Read the model definition and answer for the solid it produces. Units are mm, in the model's axes. A direction names the side the tool comes from. Round coordinates to 2 decimals unless told otherwise and drop trailing zeros. Order: outer loops, then holes, each group sorted by start corner. A loop starts at its lowest first (then second) coordinate and runs counter-clockwise, first axis right, second up. Notation, with made-up numbers: (-5.75, 13.25) - (29.25, 13.25) arc R26 ccw to (29.25, 35.25) - close; hole circle Ø10 at (17, 79). An arc over 180 degrees is marked (long way). Answer as a JSON object with one key per item and string values. Group by question number.
Q1. A cutting plane is placed at A-A on x = 0. Determine the outline of the cut face in (y, z), and give its area (3 significant figures).
Q2. A cutting plane is placed at D-D on x = 42. Determine the outline of the cut face in (y, z), and give its area (3 significant figures).
Q3. Consider line 1 (X direction, y = 280, z = -377.5); line 2 (Z direction, x = -130, y = 5.25); line 3 (Y direction, x = 130, z = -382). Determine where each line is inside the solid, lowest interval first.
Q4. A cutting plane is placed at B-B on x = -130. Count the separate pieces of the cut face and the enclosed holes in it, and give its area (3 significant figures).
Q5. Given pin 1 Ø18 at (x, y) = (-116.5, 283.5) entering from -Z; pin 2 Ø24 at (x, y) = (-130, 540) entering from -Z; pin 3 Ø1.5 at (y, z) = (152, -41) entering from -X; pin 4 Ø8 at (x, z) = (-28.5, -324) entering from +Y, each flat-ended and moving along its own axis, determine where each tip first touches the part or whether it passes through.
Q6. The mould has two halves that part along Z. Classify faces 1 (the flat face through (3, 0, 3)), 2 (the flat face through (-3, 25, -180)), 3 (the flat face through (-116, 10, 124)): pulls with the +Z half, pulls with the -Z half, needs draft (parallel to the pull), parting line crosses it, or undercut.
Q7. A tool of negligible diameter and unlimited length cuts with its end or side. For faces 4 (the flat face through (3, 230, -385)), 5 (the cylindrical face through (-136.503, 4.93, -159.287)), 6 (the cylindrical face through (100.03, 278.68, -405.07)), from which of +Z, -Z, +X, -X, +Y, -Y can it reach the whole face along a straight path? Write none if from no direction.
Solid Edge part; units mm, degrees
sketch "Sketch1" plane through (0, 0, 0) normal (1, 0, 0) x (0, 1, 0)
  line L0 (410, -260) -> (410, -410)
  line L1 (0, 0) -> (150, 0)
  arc A0 (150, 0) -> (410, -260) centre (150, -260) cw
sketch "Sketch2" plane through (0, 0, 0) normal (0, -1, 0) x (1, 0, 0)
  circle A0 centre (0, 0) radius 145
sweep "SweptProtrusion_1" add profiles "Sketch2" path "Sketch1"
sketch "Sketch3" plane through (0, 0, 0) normal (1, 0, 0) x (0, 1, 0)
  line L0 (410, -260) -> (410, -410)
  line L1 (0, 0) -> (150, 0)
  arc A0 (150, 0) -> (410, -260) centre (150, -260) cw
sketch "Sketch4" plane through (0, 0, 0) normal (0, -1, 0) x (1, 0, 0)
  circle A0 centre (0, 0) radius 130
sweep "SweptCutout_1" cut profiles "Sketch4" path "Sketch3"
sketch "Sketch5" plane through (0, 0, 0) normal (0, -1, 0) x (1, 0, 0)
  line L0 (180, 180) -> (-180, 180)
  line L1 (-180, 180) -> (-180, -180)
  line L2 (-180, -180) -> (180, -180)
  line L3 (180, -180) -> (180, 180)
  circle A0 centre (0, 0) radius 130
extrude "ExtrudedProtrusion_2" add sketch "Sketch5" against normal blind 50
sketch "Sketch6" plane through (0, 0, 0) normal (0, -1, 0) x (1, 0, 0)
  circle A0 centre (130, 130) radius 30
  circle A1 centre (-130, 130) radius 30
  circle A2 centre (-130, -130) radius 30
  circle A3 centre (130, -130) radius 30
extrude "ExtrudedCutout_1" cut sketch "Sketch6" against normal blind 10
sketch "Sketch7" plane through (0, 0, 0) normal (0, -1, 0) x (1, 0, 0)
  circle A0 centre (130, 130) radius 15
  circle A1 centre (-130, 130) radius 15
  circle A2 centre (-130, -130) radius 15
  circle A3 centre (130, -130) radius 15
extrude "ExtrudedCutout_2" cut sketch "Sketch7" against normal blind 50
mirror "Mirror1" about plane through (0, 333.8478, -76.1522) normal (0, -0.7071068, 0.7071068) of "ExtrudedProtrusion_2", "ExtrudedCutout_1", "ExtrudedCutout_2", "SweptProtrusion_1"
Result set:
{
 "1": {"outline": "(0, -180) - (50, -180) - (50, -145) - (150, -145) arc R115 cw to (265, -260) - (265, -360) - (230, -360) - (230, -410) - (590, -410) - (590, -360) - (555, -360) - (555, -260) arc R405 ccw to (150, 145) - (50, 145) - (50, 180) - (0, 180) - close", "area": "212,000 mm²"},
 "2": {"outline": "(0, -180) - (50, -180) - (50, -138.78) - (150, -138.78) arc R121.22 cw to (271.22, -260) - (271.22, -360) - (230, -360) - (230, -410) - (590, -410) - (590, -360) - (548.78, -360) - (548.78, -260) arc R398.78 ccw to (150, 138.78) - (50, 138.78) - (50, 180) - (0, 180) - close", "area": "205,000 mm²"},
 "3": {"line 1": "x = -180 to -145, -115 to 115, 145 to 180", "line 2": "z = -180 to -160, -100 to 100, 160 to 180", "line 3": "y = 230 to 265, 295 to 525, 555 to 590"},
 "4": {"separate pieces": "5", "enclosed holes": "0", "area": "107,000 mm²"},
 "5": {"pin 1": "stops at z = -400", "pin 2": "passes through", "pin 3": "stops at x = -139.3", "pin 4": "stops at y = 552.92"},
 "6": {"face 1": "needs draft", "face 2": "pulls with the -Z half", "face 3": "undercut"},
 "7": {"face 4": "-Z, +X, -X, -Y", "face 5": "-Y", "face 6": "-Z"}
}
